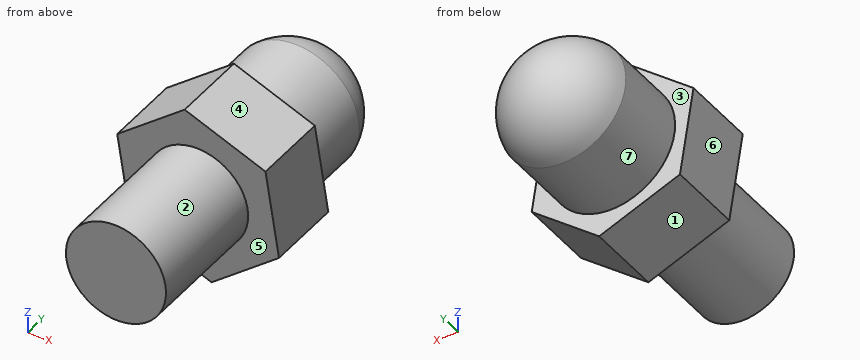
```python
from build123d import *

# Parameters (mm, degrees)
IZIM1_R                     = 2
Y_KSEKLIK_EKSTR_ZYON1_DEPTH = 5
Y_KSEKLIK_EKSTR_ZYON2_DEPTH = 3
IZIM3_R                     = 2.5
Y_KSEKLIK_EKSTR_ZYON3_DEPTH = 3
KUBBE1_FACE_RADIUS          = 2.5
KUBBE1_HEIGHT               = 2


with BuildPart() as part:
    # Çizim1 → Yükseklik-Ekstrüzyon1 (new body)
    with BuildSketch(Plane(origin=(0, 0, 0), x_dir=(1, 0, 0), z_dir=(0, 1, 0))):
        with Locations(Location((0, 0, 0), (0, 0, 270))):
            Circle(IZIM1_R)
    extrude(amount=Y_KSEKLIK_EKSTR_ZYON1_DEPTH)

    # Çizim2 → Yükseklik-Ekstrüzyon2 (add)
    with BuildSketch(Plane(origin=(0, 5, 0), x_dir=(1, 0, 0), z_dir=(0, 1, 0))):
        Polygon((2.694173307, -2.177482536), (3.232841846, 1.244481258), (0.538668539, 3.421963794), (-2.694173307, 2.177482536), (-3.232841846, -1.244481258), (-0.538668539, -3.421963794), align=None)
    extrude(amount=Y_KSEKLIK_EKSTR_ZYON2_DEPTH)

    # Çizim3 → Yükseklik-Ekstrüzyon3 (add)
    with BuildSketch(Plane(origin=(0, 8, 0), x_dir=(1, 0, 0), z_dir=(0, 1, 0))):
        with Locations(Location((0, 0, 0), (0, 0, 270))):
            Circle(IZIM3_R)
    extrude(amount=Y_KSEKLIK_EKSTR_ZYON3_DEPTH)

    # Kubbe1: a dome of height H over a round flat face of radius A is a cap of a sphere of radius (A * A + H * H) / (2 * H)
    kubbe1_r = (KUBBE1_FACE_RADIUS * KUBBE1_FACE_RADIUS + KUBBE1_HEIGHT * KUBBE1_HEIGHT) / (2 * KUBBE1_HEIGHT)
    kubbe1_base = Plane((0, 11, 0), z_dir=(0, 1, 0))
    with Locations(kubbe1_base.offset(KUBBE1_HEIGHT - kubbe1_r)):
        kubbe1_ball = Sphere(kubbe1_r, mode=Mode.PRIVATE)
    add(split(kubbe1_ball, bisect_by=kubbe1_base, keep=Keep.TOP, mode=Mode.PRIVATE))


solid = part.part
```
Geometry check sheet. Reference: the model listing, model coordinates, mm. Face numbers are marked on the shaded views. A direction names the side the tool comes from. Give positions to 0.01 mm unless a question says otherwise; leave off trailing zeros. Order: outer loops, then holes, each group sorted by start corner. A loop starts at its lowest first (then second) coordinate and runs counter-clockwise, first axis right, second up. Notation, with made-up numbers: (83.5, -35) - (92.5, -35) arc R21 cw to (92.5, -12) - close; hole circle Ø6 at (-26, 12). An arc over 180 degrees is marked (long way). Answer in a Markdown table with one row per item. Add a question column.
Q1. Tool access check on the marked faces 1, 2 and 3. Record the directions out of +Z, -Z, +X, -X, +Y, -Y that give a thin tool (end or side, any length) a straight path to the whole face; none if there is none.
Q2. Gauge pin test, flat ends, axial feed: pin 1 (3 mm diameter, centred on x = 0.5, y = 3, fed in from +Z); pin 2 (1.5 mm diameter, centred on x = -2, y = 3.5, fed in from +Z); pin 3 (1.9 mm diameter, centred on x = 0.5, z = 1, fed in from +Y). Record the tip position at first contact, or that the pin passes through.
Q3. Cross-section at D-D, the plane y = 2. Enter the section's corners in (x, z), then the cut area to 3 significant figures.
Q4. Cross-section at A-A, the plane y = 7.75. Enter the section's corners in (x, z).
Q5. Mould release check, pull along Z, two halves, no side actions. Record for the marked faces 4, 5, 6 and 7: pulls with the +Z half, pulls with the -Z half, needs draft (parallel to the pull), parting line crosses it, or undercut.
Q6. Cross-section at B-B, the plane x = -1.25. Enter the section's corners in (y, z).
Q7. Cross-section at C-C, the plane z = 0. Enter the section's corners in (x, y) (1 decimal).
Q8. Material ranges on probe 1 along Y at (x, z) = (-0.5, 2.5); probe 2 along Y at (x, z) = (-1, 0); probe 3 along X at (y, z) = (4.25, -1), recorded low to high. Write a range as from..to.
Check values:
| question | item | result |
|---|---|---|
| 1 | face 1 | -Z, -X, +Y, -Y |
| 1 | face 2 | -Y |
| 1 | face 3 | +Y |
| 2 | pin 1 | stops at z = 2 |
| 2 | pin 2 | stops at z = 1.56 |
| 2 | pin 3 | stops at y = 12.99 |
| 3 | outline | circle Ø4 at (0, 0) |
| 3 | area | 12.6 mm^2 |
| 4 | outline | (-3.23, 1.24) - (-2.69, -2.18) - (0.54, -3.42) - (3.23, -1.24) - (2.69, 2.18) - (-0.54, 3.42) - close |
| 5 | face 4 | pulls with the +Z half |
| 5 | face 5 | needs draft |
| 5 | face 6 | pulls with the -Z half |
| 5 | face 7 | parting line crosses it |
| 6 | outline | (0, -1.56) - (5, -1.56) - (5, -2.73) - (8, -2.73) - (8, -2.17) - (11, -2.17) arc R2.24 ccw to (11, 2.17) - (8, 2.17) - (8, 2.85) - (5, 2.85) - (5, 1.56) - (0, 1.56) - close |
| 7 | outline | (-3, 5) - (-2, 5) - (-2, 0) - (2, 0) - (2, 5) - (3, 5) - (3, 8) - (2.5, 8) - (2.5, 11) arc R2.6 ccw to (-2.5, 11) - (-2.5, 8) - (-3, 8) - close |
| 8 | probe 1 | y = 5..8 |
| 8 | probe 2 | y = 0..12.8 |
| 8 | probe 3 | x = -1.73..1.73 |
